Could you check a few things on this model? Use its own coordinates, in mm. A direction names the side the tool comes from. Give positions to 0.01 mm unless a question says otherwise; leave off trailing zeros. Loops run counter-clockwise (first coordinate to the right, second up) from the corner with the lowest first, then second, coordinate; pieces in that order, holes last. Notation, with made-up numbers: M 46.25,-11.75 L 93.25,-11.75 A12 cw 93.25,11.25 Z; hole C 52.5,63 d11. An arc over 180 degrees is marked long. Answer in a Markdown table with one row per item. Add a question column.
1. I'm going to push flat-ended pins straight in: pin 1 Ø2 at (x, y) = (1, -19.5) entering from -Z; pin 2 Ø1.8 at (y, z) = (0, 0) entering from -X; pin 3 Ø1.2 at (x, y) = (2, 4.5) entering from -Z. Where does each tip first touch, or does it pass through?
2. Thinking about a two-plate mould opening in Z: for faces 4 (the cylindrical face through (1.972, 0.825, 9.907)), 5 (the cylindrical face through (1.972, 8.5, 5.156)), 6 (the flat face through (4, -3, 3)), which applies, released by +Z, released by -Z, zero draft, split by the parting line, or undercut?
3. Which directions (+Z, -Z, +X, -X, +Y, -Y) give clear straight access to the entire face, cutting with the end or side of a thin tool? Please do faces 1 (the cylindrical face through (1.972, -6.461, 7.513)), 2 (the cylindrical face through (1.972, 5.148, 7.074)), 3 (the cylindrical face through (1.97, -7.53, 6.49)).
4. If we section it at A-A on z = 6.25: List the corners of the cut face in (x, y) for me.
5. If we section it at C-C on y = -19: List the corners of the cut face in (x, z) for me.
6. If we section it at B-B on x = 2.35: Count the separate pieces of the cut face and the enclosed holes in it, then the cut area to 3 significant figures.
7. I need wall thicknesses on line 1 along Y through (x, z) = (0.65, 7); line 2 along Z through (x, y) = (1.7, -1.5); line 3 along Z through (x, y) = (3.15, 9). Which ranges of each line are inside material? Lowest first, please. Write a range as from..to.
```python
from build123d import *

# Parameters (mm, degrees)
BASPROSKE_W         = 4
BASPROSKE_H         = 11
TOOTHCUT_DEPTH      = 17.062378404
TEETHCUTS_COUNT     = 20
TEETHCUTS_ANGLE     = 342
BORSKE_R            = 1.1
BORE_DEPTH          = 50.0000508
CUT_EXTRUDE_1_DEPTH = 10
EXTRUDE_1_REACH     = 38.494
SKETCH_6_W          = 4
SKETCH_6_H          = 4
FILLET_1_R          = 2
SKETCH_7_R          = 1.1
CUT_EXTRUDE_2_DEPTH = 10


with BuildPart() as part:
    # BasProSke → Base-Revolve (revolve)
    with BuildSketch(Plane(origin=(0, 0, 0), x_dir=(1, 0, 0), z_dir=(0, 1, 0)), mode=Mode.PRIVATE) as base_revolve_sk:
        with Locations((2, 5.5)):
            Rectangle(BASPROSKE_W, BASPROSKE_H)
    revolve(base_revolve_sk.sketch.rotate(Axis((-10, 0, 0), (1, 0, 0)), 180), axis=Axis((-10, 0, 0), (1, 0, 0)))

    # TooCutSke → ToothCut (cut, through all)
    with BuildSketch(Plane(origin=(0, 0, 0), x_dir=(0, 0, -1), z_dir=(1, 0, 0))):
        with BuildLine():
            ThreePointArc((0.499924007, 8.734705318), (0, 8.749), (-0.499924007, 8.734705318))
            ThreePointArc((-0.499924007, 8.734705318), (-0.824302243, 9.905497836), (-1.485192705, 10.924909509))
            ThreePointArc((-1.485192705, 10.924909509), (0, 11.0254), (1.485192705, 10.924909509))
            ThreePointArc((1.485192705, 10.924909509), (0.824302243, 9.905497836), (0.499924007, 8.734705318))
        make_face()
    toothcut = extrude(amount=TOOTHCUT_DEPTH, mode=Mode.SUBTRACT)

    # TeethCuts: ToothCut ×20 about axis
    teethcuts_axis = Axis((-10, 0, 0), (1, 0, 0))
    for i in range(1, TEETHCUTS_COUNT):
        add(toothcut.rotate(teethcuts_axis, i * TEETHCUTS_ANGLE / (TEETHCUTS_COUNT - 1)), mode=Mode.SUBTRACT)

    # BorSke → Bore (cut, symmetric)
    with BuildSketch(Plane(origin=(0, 0, 0), x_dir=(0, 0, -1), z_dir=(1, 0, 0))):
        with Locations(Location((0, 0, 0), (0, 0, 180))):
            Circle(BORSKE_R)
    extrude(amount=BORE_DEPTH, both=True, mode=Mode.SUBTRACT)

    # 草图1 → 切除-拉伸1 (cut)
    with BuildSketch(Plane(origin=(4, 0, 0), x_dir=(0, 0, -1), z_dir=(1, 0, 0))):
        with BuildLine():
            Line((0, 12.401538845), (0, 2.5))
            ThreePointArc((0, 2.5), (1.767766953, 1.767766953), (2.5, 0))
            ThreePointArc((2.5, 0), (1.767766953, -1.767766953), (0, -2.5))
            Line((0, -2.5), (0, -15.030002789))
            Line((0, -15.030002789), (15.193341894, -15.030002789))
            Line((15.193341894, -15.030002789), (15.193341894, 12.401538845))
            Line((15.193341894, 12.401538845), (0, 12.401538845))
        make_face()
    extrude(amount=-CUT_EXTRUDE_1_DEPTH, mode=Mode.SUBTRACT)

    # 草图6 → 凸台-拉伸1 (add, up to next)
    with BuildSketch(Plane(origin=(0, -24.692208515, 3.910861626), x_dir=(0, -0.1564344650402271, -0.9876883405951383), z_dir=(0, -0.9876883405951383, 0.1564344650402271)), mode=Mode.PRIVATE) as extrude_1_sk1:
        with Locations((0.210861626, 2)):
            Rectangle(SKETCH_6_W, SKETCH_6_H)
    extrude_1_tool1 = extrude(extrude_1_sk1.sketch, amount=-EXTRUDE_1_REACH, mode=Mode.PRIVATE) - part.part
    add(extrude_1_tool1.solids().sort_by_distance((2, -24.725195, 3.702596))[0])

    # 圆角1
    fillet_1_edges = [part.edges().sort_by_distance(p)[0] for p in [
        (2, -24.41232561, 5.677972738),
        (2, -25.038063471, 1.727219375),
    ]]
    fillet(fillet_1_edges, radius=FILLET_1_R - 0.0001)  # a hair under: the kernel refuses the full size

    # 草图7 → 切除-拉伸2 (cut)
    with BuildSketch(Plane(origin=(4, 0, 0), x_dir=(0, 0, -1), z_dir=(1, 0, 0))):
        with Locations((-3.389727126, -22.749817859)):
            Circle(SKETCH_7_R)
    extrude(amount=-CUT_EXTRUDE_2_DEPTH, mode=Mode.SUBTRACT)


solid = part.part
```
Results:
| question | item | result |
|---|---|---|
| 1 | pin 1 | z = 0.69 |
| 1 | pin 2 | through |
| 1 | pin 3 | z = 0 |
| 2 | face 4 | released by +Z |
| 2 | face 5 | undercut |
| 2 | face 6 | zero draft |
| 3 | face 1 | +Z, +X, -X |
| 3 | face 2 | +X, -X |
| 3 | face 3 | +X, -X, -Y |
| 4 | outline | M 0,-7.38 L 4,-7.38 L 4,7.38 L 0,7.38 Z |
| 5 | outline | M 0,0.77 L 4,0.77 L 4,4.82 L 0,4.82 Z |
| 6 | separate pieces | 1 |
| 6 | enclosed holes | 2 |
| 6 | area | 223 mm2 |
| 7 | line 1 | -7.78..-5.77, -5.25..5.25, 5.77..7.78 |
| 7 | line 2 | -2..10.9 |
| 7 | line 3 | 0.54..2.29, 3.7..5.23 |
